Autodesk Inventor part; units mm, degrees
ref_plane "YZ Plane" through (0, 0, 0) normal (1, 0, 0) x (0, 1, 0)
ref_plane "XZ Plane" through (0, 0, 0) normal (0, 1, 0) x (-1, 0, 0)
ref_plane "XY Plane" through (0, 0, 0) normal (0, 0, 1) x (1, 0, 0)
sketch "Sketch1" plane through (0, 0, 0) normal (1, 0, 0) x (0, 1, 0)
  arc A0 (1.569606, 0.130237) -> (-1.569606, 0.130237) centre (0, 0) ccw
  arc A1 (-1.996639, -5.01633) -> (1.996639, -5.01633) centre (0, -5.182) ccw
  line L0 (1.569606, 0.130237) -> (1.996639, -5.01633)
  line L1 (-1.569606, 0.130237) -> (-1.996639, -5.01633)
  arc A2 (1.996639, -5.01633) -> (-1.996639, -5.01633) centre (0, -5.182) ccw construction
  arc A3 (-1.569606, 0.130237) -> (1.569606, 0.130237) centre (0, 0) ccw construction
  line L2 (3.989789, -4.85095) -> (3.562757, 0.295617)
  arc A4 (3.562757, 0.295617) -> (-3.562757, 0.295617) centre (0, 0) ccw
  line L3 (-3.562757, 0.295617) -> (-3.989789, -4.85095)
  arc A5 (-3.989789, -4.85095) -> (3.989789, -4.85095) centre (0, -5.182) ccw
  arc A6 (3.982998, -4.769105) -> (3.569548, 0.213772) centre (3.776273, -2.277667) ccw
  arc A7 (0.970465, 1.240493) -> (3.672287, -6.776465) centre (3.776273, -2.277667) ccw construction
  arc A8 (2.870948, 2.130325) -> (0.970465, 1.240493) centre (3.776273, -2.277667) ccw construction
  arc A9 (3.672287, -6.776465) -> (2.870948, 2.130325) centre (3.776273, -2.277667) ccw
  arc A10 (1.907157, -3.93791) -> (3.982998, -4.769105) centre (3.776273, -2.277667) ccw construction
  arc A11 (3.569548, 0.213772) -> (1.907157, -3.93791) centre (3.776273, -2.277667) ccw construction
  point P0 (-1.527231, 0.384956)
  point P1 (-1.942735, -4.692312)
  point P2 (1.569795, -0.127934)
  point P3 (1.996879, -5.344741)
  dimension "d12" = 0
  dimension "d0" = 5.182
  dimension "d1" = 0
  dimension "d2" = 3.15
  dimension "d3" = 4.007
  dimension "d4" = 2
  dimension "d9" = 5
  dimension "d10" = 9
extrude "Extrusion1" add sketch "Sketch1" along normal mid plane 77 contours L0 A1 L1 A0 | A5 L3 A4 L2
extrude "Extrusion2" add sketch "Sketch1" along normal mid plane 109 contours L0 A1 L1 A0
extrude "Extrusion3" add sketch "Sketch1" along normal mid plane 5 contours L2 A6 A4 A9 A5
fillet "Fillet1" radius 3 2 edges at (0, 3.6723, -6.7765) (0, 2.8709, 2.1303)
fillet "Fillet2" radius 1 2 edges at (2.5, 6.2677, -2.0709) (-2.5, 6.2677, -2.0709)
properties part number "ChargingArm - ConnectingBrace"
Can you work these out from the model? Positions are in its coordinate system, mm. A direction names the side the tool comes from. Coordinates: 2 decimals unless noted, no trailing zeros. Loops run counter-clockwise (first coordinate to the right, second up) from the corner with the lowest first, then second, coordinate; pieces in that order, holes last.
1) Imagine slicing it at A-A on y = 0. List the corners of the cut face in (x, z) for me (1 decimal), plus the area to 3 significant figures.
2) Which directions (+Z, -Z, +X, -X, +Y, -Y) give clear straight access to the entire face, cutting with the end or side of a thin tool? Please do faces 5 (the cylindrical face through (-46.612, -0.033, 1.575)), 6 (the flat face through (38.5, -2, -3)), 7 (the flat face through (-38.5, -2, -3)), 8 (the flat face through (46.39, -1.78, -2.41)).
3) Thinking about a two-plate mould opening in Z: for faces 1 (the flat face through (-46.61, -1.78, -2.41)), 2 (the cylindrical face through (-0.035, 8.245, -1.751)), 3 (the flat face through (-2.5, 7.5, -2)), 4 (the cylindrical face through (-0.021, 6.263, -2.016)), which applies, pulls with the +Z half, pulls with the -Z half, needs draft (parallel to the pull), parting line crosses it, or undercut?
4) For pin 1 (2 mm diameter, centred on y = 6.5, z = -1, fed in from -X); pin 2 (6.5 mm diameter, centred on y = 6.5, z = -3.5, fed in from +X); pin 3 (4 mm diameter, centred on x = -41, z = -6.5, fed in from -Y), each with a flat end and sliding along its axis, tell me the tip position at first contact or that it passes through.
5) I need wall thicknesses on probe 1 along X at (y, z) = (2.25, -1); probe 2 along X at (y, z) = (4.5, 0.25); probe 3 along Y at (x, z) = (-47, 0). Which ranges of each line are inside material? Lowest first, please.
Completed:
1. outline: (-54.5, -7.2) - (-38.5, -7.2) - (-38.5, -9.2) - (38.5, -9.2) - (38.5, -7.2) - (54.5, -7.2) - (54.5, 1.6) - (38.5, 1.6) - (38.5, 3.6) - (-38.5, 3.6) - (-38.5, 1.6) - (-54.5, 1.6) - close
1. area: 1,260 mm2
2. face 5: +Z, -X
2. face 6: +X
2. face 7: -X
2. face 8: +Z, +X, -Y
3. face 1: pulls with the +Z half
3. face 2: parting line crosses it
3. face 3: needs draft
3. face 4: undercut
4. pin 1: stops at x = -2.5
4. pin 2: stops at x = 38.5
4. pin 3: stops at y = -2
5. probe 1: x = -38.5 to 38.5
5. probe 2: x = -1.99 to 1.99
5. probe 3: y = -1.58 to 1.58
